Can you work these out from the model? Positions are in its coordinate system, mm. Face numbers are marked on the shaded views. Round coordinates to 2 decimals unless told otherwise and drop trailing zeros. Order: outer loops, then holes, each group sorted by start corner. A loop starts at its lowest first (then second) coordinate and runs counter-clockwise, first axis right, second up. Notation, with made-up numbers: M 22,24.5 L 26,24.5 A17 cw 26,55.5 Z; hole C 39,78 d10. An arc over 180 degrees is marked long. One line per question, with ' | ' between items.
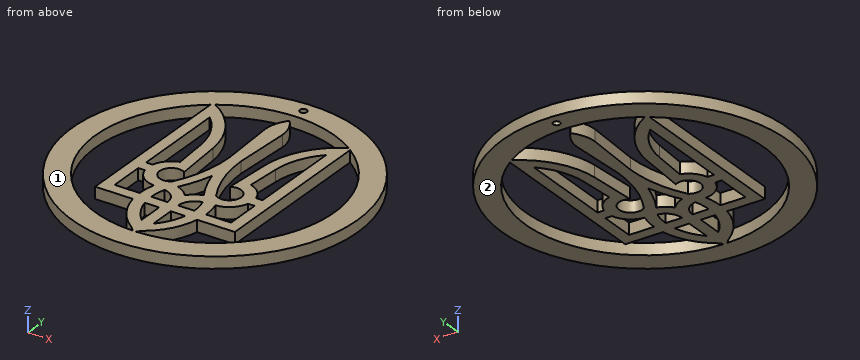
```python
from build123d import *

# Parameters (mm, degrees)
EXTRUDE_1_DEPTH = 10
SKETCH_3_R      = 122.5
SKETCH_3_R_2    = 102.5
SKETCH_3_R_3    = 3
EXTRUDE_2_DEPTH = 10


with BuildPart() as part:
    # Эскиз1 → Бобышка-Вытянуть1 (new body)
    with BuildSketch(Plane.XY):
        with BuildLine():
            Line((-60, -45), (-27.583269132, -45))
            ThreePointArc((-27.583269132, -45), (-20.06001769, -64.277376125), (-5.945767968, -79.41027067))
            ThreePointArc((-5.945767968, -79.41027067), (-2.542345747, -82.680315027), (0, -86.656865167))
            Line((0, -86.656865167), (0, -19.711115149))
            ThreePointArc((0, -19.711115149), (-5.008387109, -15.151161707), (-11.091351129, -12.172124017))
            ThreePointArc((-11.091351129, -12.172124017), (-4.677676581, 0.965070873), (0, 14.815718966))
            Line((0, 14.815718966), (0, 113.343134833))
            ThreePointArc((0, 113.343134833), (-5.562430401, 104.106601718), (-7.5, 93.5))
            Line((-7.5, 93.5), (-5, 44.25))
            ThreePointArc((-5, 44.25), (-8.525159088, 17.271181236), (-18.863936417, -7.896120801))
            ThreePointArc((-18.863936417, -7.896120801), (-34.990467135, -0.436539144), (-19.576058944, 8.401241779))
            Line((-19.576058944, 8.401241779), (-22.449472465, 49.49296956))
            ThreePointArc((-22.449472465, 49.49296956), (-33.881518529, 82.214174393), (-60, 105))
            Line((-60, 105), (-60, -45))
        make_face()
        with BuildLine():
            ThreePointArc((-26.401072965, -19.950864506), (-27.972740949, -27.40259956), (-28.5, -35))
            Line((-28.5, -35), (-50, -35))
            Line((-50, -35), (-50, -5))
            Line((-50, -5), (-44.364916731, -5))
            ThreePointArc((-44.364916731, -5), (-37.794087282, -15.372421104), (-26.401072965, -19.950864506))
        make_face(mode=Mode.SUBTRACT)
        with BuildLine():
            Line((-5, -45), (-5, -67.136427928))
            ThreePointArc((-5, -67.136427928), (-12.779082294, -56.957998409), (-17.374821937, -45))
            Line((-17.374821937, -45), (-5, -45))
        make_face(mode=Mode.SUBTRACT)
        with BuildLine():
            Line((-4.5, -35), (-18.5, -35))
            ThreePointArc((-18.5, -35), (-17.952221542, -28), (-16.322222222, -21.170419965))
            ThreePointArc((-16.322222222, -21.170419965), (-7.858362699, -25.902991945), (-4.5, -35))
        make_face(mode=Mode.SUBTRACT)
        with BuildLine():
            Line((-44.364916731, 5), (-50, 5))
            Line((-50, 5), (-50, 85.909197079))
            ThreePointArc((-50, 85.909197079), (-37.591425702, 68.515820434), (-32.355603325, 47.801370616))
            Line((-32.355603325, 47.801370616), (-30.360374841, 19.268273964))
            ThreePointArc((-30.360374841, 19.268273964), (-39.273434111, 14.009606657), (-44.364916731, 5))
        make_face(mode=Mode.SUBTRACT)
    extrude_1 = extrude(amount=EXTRUDE_1_DEPTH)

    # Зеркальное отражение1: Бобышка-Вытянуть1 across plane
    add(extrude_1.mirror(Plane(origin=(0, 0, 0), x_dir=(0, 0, 1), z_dir=(1, 0, 0))))

    # Эскиз3 → Бобышка-Вытянуть2 (add)
    with BuildSketch(Plane.XY):
        with Locations((0, 18.5)):
            Circle(SKETCH_3_R)
        with Locations((0, 18.5)):
            Circle(SKETCH_3_R_2, mode=Mode.SUBTRACT)
        with Locations((0, 131)):
            Circle(SKETCH_3_R_3, mode=Mode.SUBTRACT)
    extrude(amount=EXTRUDE_2_DEPTH)


solid = part.part
```
(1) Will these pins go through, and if not, where does the flat tip stop? pin 1 Ø2 at (x, z) = (-38, 5.5) entering from -Y; pin 2 Ø6 at (x, z) = (-46.5, 6.5) entering from +Y; pin 3 Ø3 at (y, z) = (-20.5, 3) entering from -X.
Final values:
pin 1: y = -98.28 | pin 2: y = 133.02 | pin 3: x = -116.62
(2) If we section it at B-B on x = 84.5: Please give me the cut outline in (y, z).
Final values:
outline: M -70.19,0 L -39.52,0 L -39.52,10 L -70.19,10 Z; M 76.52,0 L 107.19,0 L 107.19,10 L 76.52,10 Z
(3) If we section it at A-A on y = 0: Please give me the cut outline in (x, z) (3 decimals), plus the area to 3 significant figures.
Final values:
outline: M -121.095,0 L -100.817,0 L -100.817,10 L -121.095,10 Z; M -60,0 L -35,0 L -35,10 L -60,10 Z; M -14.78,0 L -5.079,0 L -5.079,10 L -14.78,10 Z; M 5.079,0 L 14.78,0 L 14.78,10 L 5.079,10 Z; M 35,0 L 60,0 L 60,10 L 35,10 Z; M 100.817,0 L 121.095,0 L 121.095,10 L 100.817,10 Z | area: 1,100 mm^2
(4) Thinking about a two-plate mould opening in Z: for the marked faces 1 and 2, which applies, released by +Z, released by -Z, zero draft, split by the parting line, or undercut?
Final values:
face 1: released by +Z | face 2: released by -Z
(5) If we section it at C-C on y = 37.5: Please give me the cut outline in (x, z), plus the area to 3 significant figures.
Final values:
outline: M -121.02,0 L -100.72,0 L -100.72,10 L -121.02,10 Z; M -60,0 L -50,0 L -50,10 L -60,10 Z; M -31.64,0 L -21.61,0 L -21.61,10 L -31.64,10 Z; M -5.22,0 L 5.22,0 L 5.22,10 L -5.22,10 Z; M 21.61,0 L 31.64,0 L 31.64,10 L 21.61,10 Z; M 50,0 L 60,0 L 60,10 L 50,10 Z; M 100.72,0 L 121.02,0 L 121.02,10 L 100.72,10 Z | area: 911 mm^2
(6) Please list where these lines run through material, in increasing order: probe 1 along X at (y, z) = (0, 3) (3 decimals); probe 2 along Y at (x, z) = (45.5, 2); probe 3 along Y at (x, z) = (55.5, 9.5). Write a range as [from, to].
Final values:
probe 1: [-121.095, -100.817], [-60, -35], [-14.78, -5.079], [5.079, 14.78], [35, 60], [100.817, 121.095] | probe 2: [-95.24, -73.35], [-45, -35], [-5, 5], [81.06, 95.34], [110.35, 132.24] | probe 3: [-90.71, -67.67], [-45, 102.56], [104.67, 127.71]
(7) If we section it at D-D on z = 5.5: State how many separate pieces and enclosed holes the cut face has, plus the area to 3 significant figures.
Final values:
separate pieces: 1 | enclosed holes: 13 | area: 24,500 mm^2
